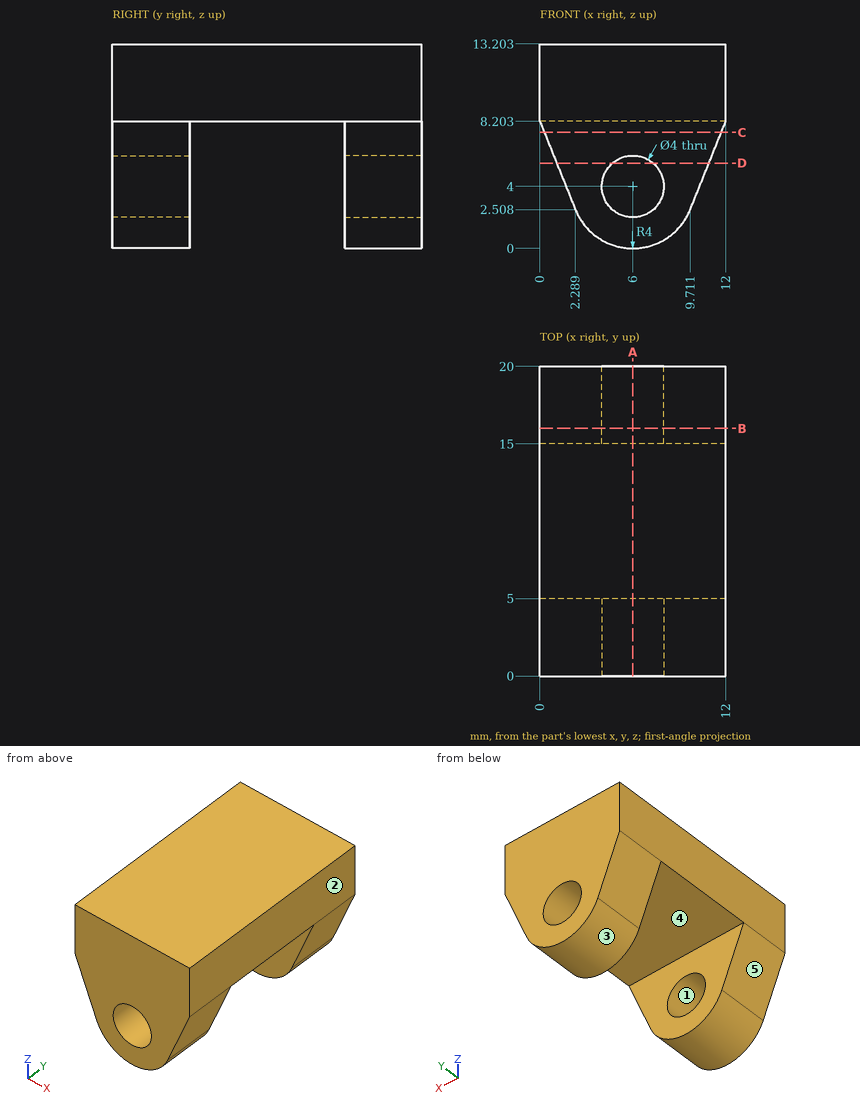
Design review of the part shown in the three views and the two pictorial views. Dimensions are in mm from the part's minimum x, y and z. A direction names the side the tool comes from. Give positions to 0.01 mm unless a question says otherwise; leave off trailing zeros. Loops run counter-clockwise (first coordinate to the right, second up) from the corner with the lowest first, then second, coordinate; pieces in that order, holes last. Notation, with made-up numbers: (-21.75, 12.5) - (25.25, 12.5) arc R15 ccw to (25.25, 35.5) - close; hole circle Ø9 at (40, -36). An arc over 180 degrees is marked (long way). Use CSV: the item, a comma, the result in double quotes. Start each with the question number.
1. Draft analysis for pull direction Z (two halves, no side actions). For the marked faces 1, 2 and 3, state which applies: released by +Z, released by -Z, zero draft, split by the parting line, or undercut.
2. Wall thickness on L1, parallel to Y at x = 2, z = 8; L2, parallel to Z at x = 1.5, y = 7.25; L3, parallel to X at y = 1.35, z = 4: over which ranges is each line inside the solid? List them lowest first.
3. Add section A-A (x = 6). State the section outline as (y, z) points, plus the area to 3 significant figures.
4. Insertion check: P1, Ø2, axis at x = 10.5, y = 7, coming from the -Z side. The pin has a flat end and moves straight along its axis. Give the tip position at first contact, or say it passes through.
5. Add section C-C (z = 7.5). State the section outline as (x, y) points.
6. Add section D-D (z = 5.5). State the section outline as (x, y) points.
7. Add section B-B (y = 16). State the section outline as (x, z) points.
8. Machinability: for the marked faces 4 and 5, which of the approach directions +Z, -Z, +X, -X, +Y, -Y give a long, thin tool a straight path to every point of the face, cutting with its end or side? Answer none if there is none.
Results found:
1,face 1,"undercut"
1,face 2,"zero draft"
1,face 3,"released by -Z"
2,L1,"y = 0 to 5, 15 to 20"
2,L2,"z = 8.2 to 13.2"
2,L3,"x = 1.69 to 4, 8 to 10.31"
3,outline,"(0, 0) - (5, 0) - (5, 2) - (0, 2) - close; (0, 6) - (5, 6) - (5, 8.2) - (15, 8.2) - (15, 6) - (20, 6) - (20, 13.2) - (0, 13.2) - close; (15, 0) - (20, 0) - (20, 2) - (15, 2) - close"
3,area,"142 mm²"
4,P1,"stops at z = 8.2"
5,outline,"(0.28, 0) - (11.72, 0) - (11.72, 5) - (0.28, 5) - close; (0.28, 15) - (11.72, 15) - (11.72, 20) - (0.28, 20) - close"
6,outline,"(1.09, 0) - (4.68, 0) - (4.68, 5) - (1.09, 5) - close; (1.09, 15) - (4.68, 15) - (4.68, 20) - (1.09, 20) - close; (7.32, 0) - (10.91, 0) - (10.91, 5) - (7.32, 5) - close; (7.32, 15) - (10.91, 15) - (10.91, 20) - (7.32, 20) - close"
7,outline,"(0, 8.2) - (2.29, 2.51) arc R4 ccw to (9.71, 2.51) - (12, 8.2) - (12, 13.2) - (0, 13.2) - close; hole circle Ø4 at (6, 4)"
8,face 4,"-Z, +X, -X"
8,face 5,"-Z, -X, +Y, -Y"
